```python
from build123d import *

# Parameters (mm, degrees)
SKETCH_1_W                 = 60
SKETCH_1_H                 = 30
EXTRUDE_1_DEPTH            = 7
SKETCH_2_W                 = 59
SKETCH_2_H                 = 29
EXTRUDE_2_DEPTH            = 2
SKETCH_3_W                 = 57
SKETCH_3_H                 = 27
CUT_EXTRUDE_1_DEPTH        = 7.5
SKETCH_4_W                 = 44
SKETCH_4_H                 = 1
EXTRUDE_3_DEPTH            = 0.5
CHAMFER_1_SIZE             = 0.5
CHAMFER_1_OF_MIRROR_1_SIZE = 0.5
CUT_EXTRUDE_2_DEPTH        = 5
FILLET_1_R                 = 0.2


with BuildPart() as part:
    # 草图1 → 凸台-拉伸1 (new body)
    with BuildSketch(Plane(origin=(0, 0, 0), x_dir=(1, 0, 0), z_dir=(0, 1, 0))):
        Rectangle(SKETCH_1_W, SKETCH_1_H)
    extrude(amount=EXTRUDE_1_DEPTH)

    # 草图2 → 凸台-拉伸2 (add)
    with BuildSketch(Plane(origin=(0, 7, 0), x_dir=(1, 0, 0), z_dir=(0, 1, 0))):
        Rectangle(SKETCH_2_W, SKETCH_2_H)
    extrude(amount=EXTRUDE_2_DEPTH)

    # 草图3 → 切除-拉伸1 (cut)
    with BuildSketch(Plane(origin=(0, 9, 0), x_dir=(1, 0, 0), z_dir=(0, 1, 0))):
        Rectangle(SKETCH_3_W, SKETCH_3_H)
    extrude(amount=-CUT_EXTRUDE_1_DEPTH, mode=Mode.SUBTRACT)

    # 草图4 → 凸台-拉伸3 (add)
    with BuildSketch(Plane(origin=(0, 0, -14.5), x_dir=(-1, 0, 0), z_dir=(0, 0, -1))):
        with Locations((0, 8.5)):
            Rectangle(SKETCH_4_W, SKETCH_4_H)
    extrude_3 = extrude(amount=EXTRUDE_3_DEPTH)

    # 倒角1
    chamfer_1_edges = [part.edges().sort_by_distance(p)[0] for p in [
        (0, 9, -15),
    ]]
    chamfer(chamfer_1_edges, length=CHAMFER_1_SIZE)

    # 镜向1: 凸台-拉伸3 across plane
    add(extrude_3.mirror(Plane.XY))

    # 倒角1 of 镜向1
    chamfer_1_of_mirror_1_edges = [part.edges().sort_by_distance(p)[0] for p in [
        (0, 9, 15),
    ]]
    chamfer(chamfer_1_of_mirror_1_edges, length=CHAMFER_1_OF_MIRROR_1_SIZE)

    # 草图5 → 切除-拉伸2 (cut)
    with BuildSketch(Plane(origin=(0, 9, 0), x_dir=(1, 0, 0), z_dir=(0, 1, 0))):
        Polygon((30, 0), (30, 1.5), (28.5, 1.5), (28.5, -1.5), (30, -1.5), align=None)
    extrude(amount=-CUT_EXTRUDE_2_DEPTH, mode=Mode.SUBTRACT)

    # 圆角1
    fillet_1_edges = [part.edges().sort_by_distance(p)[0] for p in [
        (0, 7, 15),
        (30, 7, 8.25),
        (0, 7, -15),
        (30, 0, 0),
        (0, 0, 15),
        (-30, 0, 0),
        (0, 0, -15),
        (-30, 7, 0),
        (30, 3.5, -15),
        (30, 3.5, 15),
        (-30, 3.5, 15),
        (-30, 3.5, -15),
        (30, 7, -8.25),
        (30, 5.5, 1.5),
        (30, 4, 0),
        (30, 5.5, -1.5),
    ]]
    fillet(fillet_1_edges, radius=FILLET_1_R)


solid = part.part
```
Source: CAD feature listing. Evaluate the final solid. Frame: model axes, mm. A direction names the side the tool comes from. Give positions to 0.01 mm unless a question says otherwise; leave off trailing zeros. Write each loop counter-clockwise with the first axis right and the second up, starting at its lowest first coordinate (ties: lowest second). Pieces come first, ordered by that corner, then holes. Notation, with made-up numbers: (8, 5) - (50, 5) arc R21 cw to (50, 19) - close; hole circle Ø9 at (39.5, 61.5). An arc over 180 degrees is marked (long way). One line per item, written item: value. Start each with the question number.
Q1. Section query A-A, the plane z = -4.25. Return the cut outline in (x, y).
Q2. Material intervals for probe 1 along Z at (x, y) = (-16, 3.25); probe 2 along X at (y, z) = (7.75, 6.75); probe 3 along X at (y, z) = (1.75, -4.5), sorted ascending. Write a range as from..to.
Q3. Draft query along X for faces 4 (the face through (29, 7, 1.5)), 5 (the face through (28.5, 3.6, 0.2)), 6 (the face through (30, 3, 0)). Return one class per face: +X half, -X half, draft (parallel to the pull), parting line (faces both ways), or undercut.
Q4. First-contact query: pin 1 Ø1.5 at (x, z) = (7.5, 4) entering from +Y; pin 2 Ø0.6 at (y, z) = (8, 2.5) entering from -X; pin 3 Ø0.6 at (y, z) = (8.5, -15) entering from +X. Flat tips, straight axial feed; report the tip coordinate or a pass-through.
Q5. Set-up query: faces 1 (the face through (29.5, 8, -8)), 2 (the face through (0, 5, -13.5)), 3 (the face through (29, 4, 0)). Return all of +Z, -Z, +X, -X, +Y, -Y with unobstructed straight access to the full face (end or side cutting, diameter ignored); none if empty.
Q6. Section query B-B, the plane x = -17. Return the cut outline in (y, z), then the cut area to 3 significant figures.
Q7. Section query D-D, the plane y = 6. Return the cut outline in (x, z).
Q8. Section query C-C, the plane y = 3. Return the cut outline in (x, z), then the cut area to 3 significant figures.
Answer:
1. outline: (-30, 0.2) arc R0.2 ccw to (-29.8, 0) - (29.8, 0) arc R0.2 ccw to (30, 0.2) - (30, 6.8) arc R0.2 ccw to (29.8, 7) - (29.5, 7) - (29.5, 9) - (28.5, 9) - (28.5, 1.5) - (-28.5, 1.5) - (-28.5, 9) - (-29.5, 9) - (-29.5, 7) - (-29.8, 7) arc R0.2 ccw to (-30, 6.8) - close
2. probe 1: z = -15..-13.5, 13.5..15
2. probe 2: x = -29.5..-28.5, 28.5..29.5
2. probe 3: x = -30..-28.5, 28.5..30
3. face 4: draft
3. face 5: undercut
3. face 6: +X half
4. pin 1: stops at y = 1.5
4. pin 2: stops at x = -29.5
4. pin 3: stops at x = 22
5. face 1: +Z, -Z, +X, +Y
5. face 2: +Y
5. face 3: +X, +Y
6. outline: (0, -14.8) arc R0.2 ccw to (0.2, -15) - (6.8, -15) arc R0.2 ccw to (7, -14.8) - (7, -14.5) - (8, -14.5) - (8, -15) - (8.5, -15) - (9, -14.5) - (9, -13.5) - (1.5, -13.5) - (1.5, 13.5) - (9, 13.5) - (9, 14.5) - (8.5, 15) - (8, 15) - (8, 14.5) - (7, 14.5) - (7, 14.8) arc R0.2 ccw to (6.8, 15) - (0.2, 15) arc R0.2 ccw to (0, 14.8) - close
6. area: 66.2 mm2
7. outline: (-30, -14.8) arc R0.2 ccw to (-29.8, -15) - (29.8, -15) arc R0.2 ccw to (30, -14.8) - (30, -1.7) arc R0.2 ccw to (29.8, -1.5) - (28.5, -1.5) - (28.5, -13.5) - (-28.5, -13.5) - (-28.5, 13.5) - (28.5, 13.5) - (28.5, 1.5) - (29.8, 1.5) arc R0.2 ccw to (30, 1.7) - (30, 14.8) arc R0.2 ccw to (29.8, 15) - (-29.8, 15) arc R0.2 ccw to (-30, 14.8) - close
8. outline: (-30, -14.8) arc R0.2 ccw to (-29.8, -15) - (29.8, -15) arc R0.2 ccw to (30, -14.8) - (30, 14.8) arc R0.2 ccw to (29.8, 15) - (-29.8, 15) arc R0.2 ccw to (-30, 14.8) - close; hole (-28.5, -13.5) - (28.5, -13.5) - (28.5, 13.5) - (-28.5, 13.5) - close
8. area: 261 mm2
